Can you work these out from the model? Positions are in its coordinate system, mm. A direction names the side the tool comes from. Give positions to 0.01 mm unless a question says otherwise; leave off trailing zeros. Write each loop counter-clockwise with the first axis right and the second up, starting at its lowest first coordinate (ties: lowest second). Pieces come first, ordered by that corner, then holes. Notation, with made-up numbers: (-30.75, -12.75) -> (-16.75, -12.75) arc R31 cw to (-16.75, 13.25) -> close; hole circle Ø7 at (89, 76). An arc over 180 degrees is marked (long way). One line per item, written item: value.
from build123d import *

# Parameters (mm, degrees)
F0_R     = 6.35
F1_DEPTH = 279.4
F2_R     = 6.35
F2_R_2   = 3.175
F3_DEPTH = 25.4
F4_R     = 3.175
F5_DEPTH = 25.4


with BuildPart() as f1:
    # F0 (on Front) → F1 (new body)
    with BuildSketch(Plane.XZ):
        Circle(F0_R)
    extrude(amount=F1_DEPTH)

    # F2 (on face) → F3 (cut)
    with BuildSketch(Plane(origin=(0, 0, 0), x_dir=(-1, 0, 0), z_dir=(0, 1, 0))):
        Circle(F2_R)
        Circle(F2_R_2, mode=Mode.SUBTRACT)
    extrude(amount=-F3_DEPTH, mode=Mode.SUBTRACT)

    # F4 (on face) → F5 (cut)
    with BuildSketch(Plane.XZ.offset(279.4)):
        Circle(F4_R)
    extrude(amount=-F5_DEPTH, mode=Mode.SUBTRACT)


solid = f1.part
1) We'd pull the mould along X, two halves only. Please class faces 1 (the face through (0, 0, 0)), 2 (the face through (-0.69, -266.88, -3.1)), 3 (the face through (-1.38, -150.62, -6.2)): released by +X, released by -X, zero draft, split by the parting line, or undercut.
Answer list:
face 1: zero draft
face 2: undercut
face 3: split by the parting line
2) For faces 4 (the face through (0, -254, 0)), 5 (the face through (0.69, -12.52, -3.1)), 6 (the face through (-2, -279.4, 3)), which set-ups out of +Z, -Z, +X, -X, +Y, -Y let a thin tool reach every point of the face, with its end or its side?
Answer list:
face 4: -Y
face 5: +Y
face 6: +Z, -Z, +X, -X, -Y
3) If we section it at C-C (y = -172.5): Write out the boundary of the cut face in (x, z).
Answer list:
outline: circle Ø12.7 at (0, 0)
4) Will these pins go through, and if not, where does the flat tip stop? pin 1 (3 mm diameter, centred on y = -242, z = 3, fed in from -X); pin 2 (3 mm diameter, centred on y = -220.5, z = 2, fed in from +X); pin 3 (1.9 mm diameter, centred on x = 1, z = 0.5, fed in from -Y); pin 4 (3 mm diameter, centred on y = -169.5, z = 1.5, fed in from -X).
Answer list:
pin 1: stops at x = -6.17
pin 2: stops at x = 6.33
pin 3: stops at y = -254
pin 4: stops at x = -6.35
5) If we section it at B-B (x = 0): Write out the boundary of the cut face in (y, z) (3 decimals).
Answer list:
outline: (-279.4, -6.35) -> (-25.4, -6.35) -> (-25.4, -3.175) -> (0, -3.175) -> (0, 3.175) -> (-25.4, 3.175) -> (-25.4, 6.35) -> (-279.4, 6.35) -> (-279.4, 3.175) -> (-254, 3.175) -> (-254, -3.175) -> (-279.4, -3.175) -> close
6) I need wall thicknesses on L1, parallel to Z at x = 0, y = -264 (3 decimals); L2, parallel to X at y = -64.5, z = -0.25; L3, parallel to Y at x = 1.5, z = -1.75. Which ranges of each line are inside material? Lowest first, please.
Answer list:
L1: z = -6.35 to -3.175, 3.175 to 6.35
L2: x = -6.35 to 6.35
L3: y = -254 to 0
7) If we section it at A-A (z = 0): Write out the boundary of the cut face in (x, y) (3 decimals), and give its area (3 significant figures).
Answer list:
outline: (-6.35, -279.4) -> (-3.175, -279.4) -> (-3.175, -254) -> (3.175, -254) -> (3.175, -279.4) -> (6.35, -279.4) -> (6.35, -25.4) -> (3.175, -25.4) -> (3.175, 0) -> (-3.175, 0) -> (-3.175, -25.4) -> (-6.35, -25.4) -> close
area: 3,230 mm^2
